Study the drawing (mm; zero at the part's minimum x, y, z) and answer. A direction names the side the tool comes from. Round coordinates to 2 decimals unless told otherwise and drop trailing zeros. Write each loop counter-clockwise with the first axis right and the second up, starting at its lowest first coordinate (ties: lowest second). Pieces come first, ordered by that corner, then holes. Notation, with made-up numbers: (36.5, 19.5) - (46.5, 19.5) arc R14 cw to (46.5, 25.5) - close; hole circle Ø11 at (31.25, 33). An arc over 180 degrees is marked (long way). Use one line per item in the form item = value. Start each with the question number.
1) For the marked faces 4 and 5, determine the directions among +Z, -Z, +X, -X, +Y, -Y from which every point of the face is accessible in a straight line to the end or side of a thin tool.
2) For a pull along Y with two mould halves and no side action, classify the marked faces 1, 2 and 3 as released by +Y, released by -Y, zero draft, split by the parting line, or undercut.
3) The part is cut by section B-B, the plane z = 2. Give the vertices of the cut face in (x, y).
4) The part is cut by section A-A, the plane x = 6. Give the vertices of the cut face in (y, z), plus the area to 3 significant figures.
5) Each of these flat-tipped pins is pushed along its axis until it touches: pin 1 (3 mm diameter, centred on x = 5, y = 4, fed in from +Z); pin 2 (2 mm diameter, centred on x = 2, z = 2.5, fed in from +Y) (1 decimal); pin 3 (2 mm diameter, centred on x = 8.5, z = 1, fed in from +Y); pin 4 (0.5 mm diameter, centred on x = 13, z = 2, fed in from +Y). Where does it stop, or does it pass through?
6) The part is cut by section C-C, the plane y = 9.5. Give the vertices of the cut face in (x, z).
7) The part is cut by section D-D, the plane y = 6.5. Give the vertices of the cut face in (x, z) (1 decimal).
8) Consider line 1 along Y through (x, z) = (6, 1.1); line 2 along Y through (x, z) = (3.75, 2.4) (1 decimal); line 3 along X through (y, z) = (1.5, 1.2). Determine where each line is inside the solid, lowest interval first. Write a range as from..to.
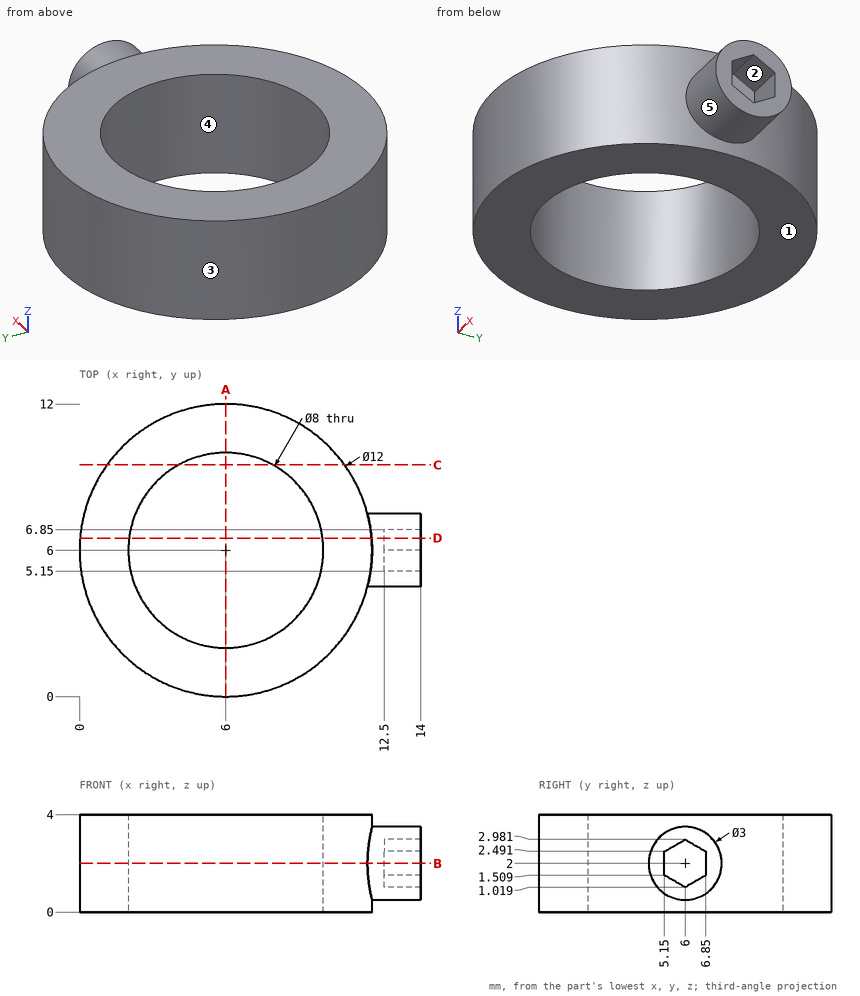
Geometry results:
q1.face_4 = +Z, -Z
q1.face_5 = +X
q2.face_1 = zero draft
q2.face_2 = undercut
q2.face_3 = split by the parting line
q3.outline = (11.81, 4.5) - (14, 4.5) - (14, 5.15) - (12.5, 5.15) - (12.5, 6.85) - (14, 6.85) - (14, 7.5) - (11.81, 7.5) arc R6 ccw (long way) to start; hole circle Ø8 at (6, 6)
q4.outline = (0, 0) - (2, 0) - (2, 4) - (0, 4) - close; (10, 0) - (12, 0) - (12, 4) - (10, 4) - close
q4.area = 16.0 mm2
q5.pin_1 = through
q5.pin_2 = 11.2
q5.pin_3 = 11.81
q5.pin_4 = 7.5
q6.outline = (1.13, 0) - (4.06, 0) - (4.06, 4) - (1.13, 4) - close; (7.94, 0) - (10.87, 0) - (10.87, 4) - (7.94, 4) - close
q7.outline = (0, 0) - (2, 0) - (2, 4) - (0, 4) - close; (10, 0) - (12, 0) - (12, 0.6) - (14, 0.6) - (14, 1.3) - (12.5, 1.3) - (12.5, 2.7) - (14, 2.7) - (14, 3.4) - (12, 3.4) - (12, 4) - (10, 4) - close
q8.line_1 = 0..2, 10..12
q8.line_2 = 0.4..2.7, 9.3..11.6
q8.line_3 = 2.03..9.97
